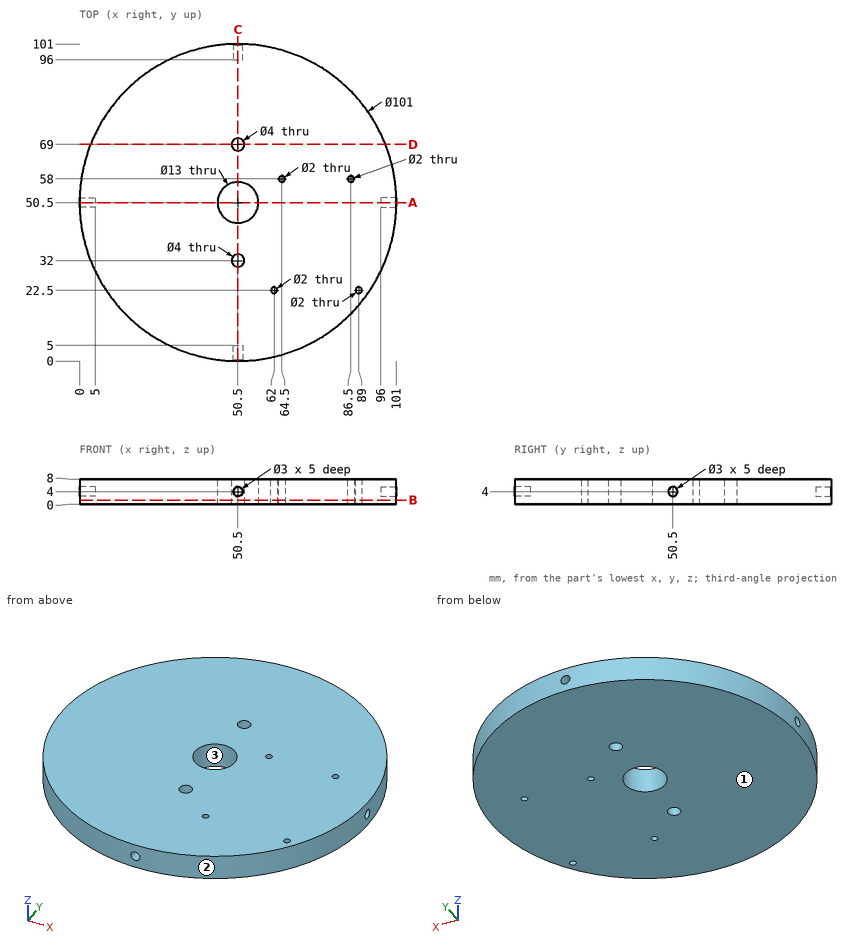
Check sheet for the drawn part. Datum: minimum x, y, z corner. Units: mm. Give positions to 0.01 mm unless a question says otherwise; leave off trailing zeros. Loops run counter-clockwise (first coordinate to the right, second up) from the corner with the lowest first, then second, coordinate; pieces in that order, holes last.
1) Sectioned sample at A-A, the plane y = 50.5. Enter the section's corners in (x, z).
2) Thickness scan on line 1 along Y through (x, z) = (62, 5.75); line 2 along Y through (x, z) = (64.5, 5.5); line 3 along X through (y, z) = (22, 5). Record the ranges inside material, lowest first.
3) Depth check by flat-ended pin: pin 1 Ø2.5 at (y, z) = (50.5, 4) entering from +X; pin 2 Ø4 at (y, z) = (78, 6.5) entering from +X; pin 3 Ø1 at (x, z) = (71.5, 3) entering from +Y. Enter the tip coordinate at first touch or a pass-through.
4) Sectioned sample at D-D, the plane y = 69. Enter the section's corners in (x, z).
5) Sectioned sample at B-B, the plane z = 1.25. Enter the section's corners in (x, y).
6) Sectioned sample at C-C, the plane x = 50.5. Enter the section's corners in (y, z).
7) Draft check along Y on the marked faces 1, 2 and 3. Enter one of: pulls with the +Y half, pulls with the -Y half, needs draft (parallel to the pull), parting line crosses it, or undercut.
Answers:
1. outline: (0, 0) - (44, 0) - (44, 8) - (0, 8) - (0, 5.5) - (5, 5.5) - (5, 2.5) - (0, 2.5) - close; (57, 0) - (101, 0) - (101, 2.5) - (96, 2.5) - (96, 5.5) - (101, 5.5) - (101, 8) - (57, 8) - close
2. line 1: y = 1.33 to 21.5, 23.5 to 99.67
2. line 2: y = 1.98 to 57, 59 to 99.02
2. line 3: x = 8.81 to 61.13, 62.87 to 88.13, 89.87 to 92.19
3. pin 1: stops at x = 96
3. pin 2: stops at x = 94.09
3. pin 3: stops at y = 96.65
4. outline: (3.51, 0) - (48.5, 0) - (48.5, 8) - (3.51, 8) - close; (52.5, 0) - (97.49, 0) - (97.49, 8) - (52.5, 8) - close
5. outline: circle Ø101 at (50.5, 50.5); hole circle Ø13 at (50.5, 50.5); hole circle Ø4 at (50.5, 32); hole circle Ø4 at (50.5, 69); hole circle Ø2 at (62, 22.5); hole circle Ø2 at (64.5, 58); hole circle Ø2 at (86.5, 58); hole circle Ø2 at (89, 22.5)
6. outline: (0, 0) - (30, 0) - (30, 8) - (0, 8) - (0, 5.5) - (5, 5.5) - (5, 2.5) - (0, 2.5) - close; (34, 0) - (44, 0) - (44, 8) - (34, 8) - close; (57, 0) - (67, 0) - (67, 8) - (57, 8) - close; (71, 0) - (101, 0) - (101, 2.5) - (96, 2.5) - (96, 5.5) - (101, 5.5) - (101, 8) - (71, 8) - close
7. face 1: needs draft
7. face 2: parting line crosses it
7. face 3: undercut
